from build123d import *

# Parameters (mm, degrees)
BOSS_EXTRUDE1_DEPTH = 20
SKETCH2_R           = 2
CUT_EXTRUDE1_DEPTH  = 233.365552524
CUT_EXTRUDE2_START  = -15
SKETCH2_3_R         = 2
CUT_EXTRUDE2_DEPTH  = 5
SKETCH2_4_R         = 2
CUT_EXTRUDE3_DEPTH  = 5


with BuildPart() as part:
    # Sketch1 → Boss-Extrude1 (new body)
    with BuildSketch(Plane(origin=(0, 0, 0), x_dir=(1, 0, 0), z_dir=(0, 1, 0))):
        Polygon((0, 155), (0, 175), (46.891108675, 175), (128.108891325, 128.108891325), (151.554445662, 87.5), (134.233937587, 77.5), (113.467875173, 113.467875173), (41.532124827, 155), align=None)
    extrude(amount=BOSS_EXTRUDE1_DEPTH)

    # Sketch2 → Cut-Extrude1 (cut, through all)
    with BuildSketch(Plane(origin=(0, 20, 0), x_dir=(1, 0, 0), z_dir=(0, 1, 0))):
        with Locations(Location((7.5, 165, 0), (0, 0, 270))):
            Circle(SKETCH2_R)
        with Locations(Location((22.5, 165, 0), (0, 0, 270))):
            Circle(SKETCH2_R)
        with Locations(Location((131.644191624, 101.985571585, 0), (0, 0, 270))):
            Circle(SKETCH2_R)
        with Locations(Location((139.144191624, 88.995190528, 0), (0, 0, 90))):
            Circle(SKETCH2_R)
    extrude(amount=-CUT_EXTRUDE1_DEPTH, mode=Mode.SUBTRACT)

    # Sketch2<3> → Cut-Extrude2 (cut)
    # profile 1 of 2: a face of its own
    with BuildSketch(Plane(origin=(0, 20, 0), x_dir=(1, 0, 0), z_dir=(0, 1, 0)).offset(CUT_EXTRUDE2_START)):
        Polygon((3.8, 167.136195996), (3.8, 162.863804004), (7.5, 160.727608008), (11.2, 162.863804004), (11.2, 167.136195996), (7.5, 169.272391992), align=None)
        with Locations(Location((7.5, 165, 0), (0, 0, 270))):
            Circle(SKETCH2_3_R, mode=Mode.SUBTRACT)
    # profile 2 of 2: a face of its own
    with BuildSketch(Plane(origin=(0, 20, 0), x_dir=(1, 0, 0), z_dir=(0, 1, 0)).offset(CUT_EXTRUDE2_START)):
        Polygon((26.2, 162.863804004), (26.2, 167.136195996), (22.5, 169.272391992), (18.8, 167.136195996), (18.8, 162.863804004), (22.5, 160.727608008), align=None)
        with Locations(Location((22.5, 165, 0), (0, 0, 270))):
            Circle(SKETCH2_3_R, mode=Mode.SUBTRACT)
    extrude(amount=-CUT_EXTRUDE2_DEPTH, mode=Mode.SUBTRACT)

    # Sketch2<4> → Cut-Extrude3 (cut)
    # profile 1 of 2: a face of its own
    with BuildSketch(Plane(origin=(0, 20, 0), x_dir=(1, 0, 0), z_dir=(0, 1, 0))):
        Polygon((135.344191624, 104.121767581), (135.344191624, 99.849375589), (131.644191624, 97.713179593), (127.944191624, 99.849375589), (127.944191624, 104.121767581), (131.644191624, 106.257963577), align=None)
        with Locations(Location((131.644191624, 101.985571585, 0), (0, 0, 270))):
            Circle(SKETCH2_4_R, mode=Mode.SUBTRACT)
    # profile 2 of 2: a face of its own
    with BuildSketch(Plane(origin=(0, 20, 0), x_dir=(1, 0, 0), z_dir=(0, 1, 0))):
        Polygon((135.444191624, 86.858994532), (135.444191624, 91.131386524), (139.144191624, 93.26758252), (142.844191624, 91.131386524), (142.844191624, 86.858994532), (139.144191624, 84.722798536), align=None)
        with Locations(Location((139.144191624, 88.995190528, 0), (0, 0, 270))):
            Circle(SKETCH2_4_R, mode=Mode.SUBTRACT)
    extrude(amount=-CUT_EXTRUDE3_DEPTH, mode=Mode.SUBTRACT)


solid = part.part
Design review of the part built by this model. Coordinates are the model's own, in mm. A direction names the side the tool comes from. Give positions to 0.01 mm unless a question says otherwise; leave off trailing zeros. Write each loop counter-clockwise with the first axis right and the second up, starting at its lowest first coordinate (ties: lowest second). Pieces come first, ordered by that corner, then holes. Notation, with made-up numbers: M -40,59 L 6,59 A24 cw 6,97 Z; hole C -32.75,18 d2. An arc over 180 degrees is marked long. Return JSON: item names as keys, results as strings. Group by question number.
Item 1: Clearance check with flat-ended pins moving along their axes: pin 1 Ø1.3 at (y, z) = (2.5, -164.5) entering from -X; pin 2 Ø4 at (x, y) = (101, 16) entering from -Z; pin 3 Ø4.5 at (y, z) = (2.5, -165) entering from +X; pin 4 Ø2 at (y, z) = (18, -89.5) entering from -X. State where each tip first meets the part, or that it passes through.
Item 2: The part is to be moulded in two halves that separate along X. For faces 4 (the flat face through (135.444, 18, -89)), 5 (the flat face through (76, 20, -137)), 6 (the flat face through (123.996, 9.86, -95.232)), say which applies: pulls with the +X half, pulls with the -X half, needs draft (parallel to the pull), parting line crosses it, or undercut.
Item 3: Wall thickness on line 1 along X through (y, z) = (13.25, -165); line 2 along Y through (x, z) = (138.5, -86); line 3 along Z through (x, y) = (132, 1.25): over which ranges is each line inside the solid? List them lowest first.
Item 4: Take a section at A-A (y = 13.25). Give the boundary of the cut face in (x, z).
Item 5: Take a section at B-B (z = -165). Give the boundary of the cut face in (x, y).
Item 6: Take a section at C-C (z = -115). Give the boundary of the cut face in (x, y).
Item 7: Tool access review of faces 1 (the flat face through (139.668, 9.86, -108.089)), 2 (the flat face through (9.32, 2.54, -161.78)), 3 (the flat face through (137.32, 17.535, -85.776)): name each direction out of +Z, -Z, +X, -X, +Y, -Y from which nothing blocks a thin tool from reaching the whole face with its end or side.
Return value:
{
 "1": {"pin 1": "stops at x = 0", "pin 2": "stops at z = -144.91", "pin 3": "stops at x = 68.11", "pin 4": "stops at x = 126.73"},
 "2": {"face 4": "undercut", "face 5": "needs draft", "face 6": "pulls with the -X half"},
 "3": {"line 1": "x = 0 to 5.5, 9.5 to 20.5, 24.5 to 64.21", "line 2": "y = 0 to 15", "line 3": "z = -121.37 to -103.95, -100.02 to -81.37"},
 "4": {"outline": "M 0,-175 L 46.89,-175 L 128.11,-128.11 L 151.55,-87.5 L 134.23,-77.5 L 113.47,-113.47 L 41.53,-155 L 0,-155 Z; hole C 7.5,-165 d4; hole C 22.5,-165 d4; hole C 131.64,-101.99 d4; hole C 139.14,-89 d4"},
 "5": {"outline": "M 0,0 L 3.8,0 L 3.8,5 L 5.5,5 L 5.5,20 L 0,20 Z; M 9.5,5 L 11.2,5 L 11.2,0 L 18.8,0 L 18.8,5 L 20.5,5 L 20.5,20 L 9.5,20 Z; M 24.5,5 L 26.2,5 L 26.2,0 L 64.21,0 L 64.21,20 L 24.5,20 Z"},
 "6": {"outline": "M 110.81,0 L 135.68,0 L 135.68,20 L 110.81,20 Z"},
 "7": {"face 1": "-Z, +X, +Y, -Y", "face 2": "-Y", "face 3": "+Y"}
}
